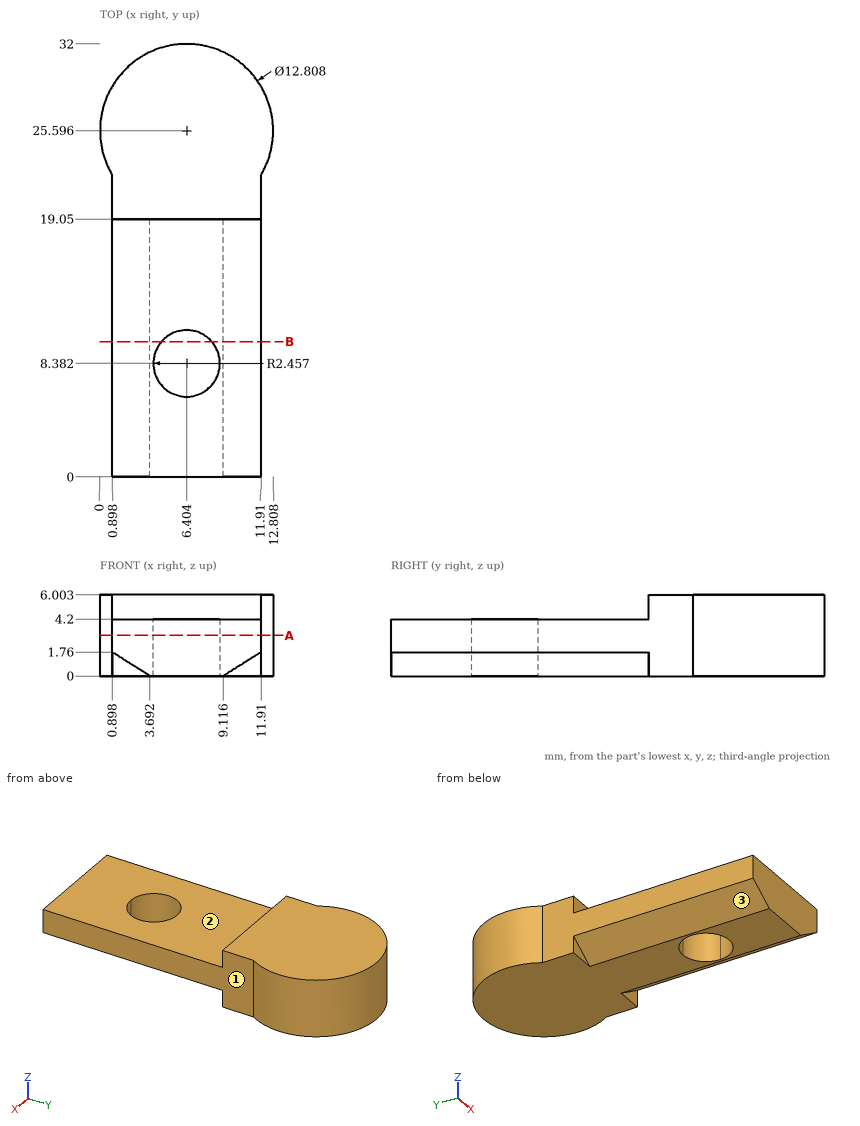
Input: dimensioned drawing with shaded views. Units: mm. Origin: part minimum x, y, z. A direction names the side the tool comes from. Give positions to 0.01 mm unless a question says otherwise; leave off trailing zeros. Loops run counter-clockwise (first coordinate to the right, second up) from the corner with the lowest first, then second, coordinate; pieces in that order, holes last. Notation, with made-up numbers: M 32,20 L 44,20 A16 ccw 44,37 Z; hole C 80,61 d7. An arc over 180 degrees is marked long. Put each result on its own line as item: value. Start each with the question number.
1) Contact query for flat-ended pins moving along their axis: pin 1 (0.9 mm diameter, centred on x = 6, z = 5.5, fed in from -Y); pin 2 (3 mm diameter, centred on y = 13, z = 2, fed in from +X); pin 3 (5.5 mm diameter, centred on x = 8, y = 11, fed in from +Z). Output: stop coordinate, or through.
2) Cut plane B-B (y = 10). Output: boundary loops of the cut face in (x, z) (1 decimal), then the cut area to 3 significant figures.
3) Ray query, line 1 along Y through (x, z) = (6.25, 3) (1 decimal); line 2 along Y through (x, z) = (6.5, 4.25); line 3 along X through (y, z) = (17, 3.75). Return the intervals inside material, ascending.
4) Cut plane A-A (z = 3). Output: boundary loops of the cut face in (x, y) (1 decimal).
5) Access query for the marked faces 1, 2 and 3. Directions: +Z, -Z, +X, -X, +Y, -Y. A direction counts if a zero-diameter tool reaches every point of the face in a straight line with its end or side. Return the directions, or none.
Verdict:
1. pin 1: y = 19.05
1. pin 2: x = 11.91
1. pin 3: z = 4.2
2. outline: M 0.9,1.8 L 3.7,0 L 4.6,0 L 4.6,4.2 L 0.9,4.2 Z; M 8.3,0 L 9.1,0 L 11.9,1.8 L 11.9,4.2 L 8.3,4.2 Z
2. area: 25.8 mm2
3. line 1: 0 to 5.9, 10.8 to 32
3. line 2: 19.05 to 32
3. line 3: 0.9 to 11.91
4. outline: M 0.9,0 L 11.9,0 L 11.9,22.3 A6.4 ccw long 0.9,22.3 Z; hole M 6.4,5.9 A2.5 ccw 8.9,8.4 A2.5 ccw long Z
5. face 1: +Z, -Z, +X, -Y
5. face 2: +Z, +X, -X, -Y
5. face 3: -Z, -X, -Y
